from build123d import *

# Parameters (mm, degrees)
SKETCH1_W                              = 14
SKETCH1_H                              = 15
BOSS_EXTRUDE1_DEPTH                    = 50
CBORE_FOR_M6_HEX_HEAD_BOLT1_AT_2_COUNT = 2
CBORE_FOR_M6_HEX_HEAD_BOLT1_AT_2_PITCH = 20


with BuildPart() as part:
    # Sketch1 → Boss-Extrude1 (new body)
    with BuildSketch(Plane.XY):
        Rectangle(SKETCH1_W, SKETCH1_H)
    extrude(amount=BOSS_EXTRUDE1_DEPTH)

    # Sketch3 → CBORE for M6 Hex Head Bolt1 (revolve, cut)
    with BuildSketch(Plane(origin=(-7, 0, 10), x_dir=(0, 0, 1), z_dir=(0, 1, 0))):
        Polygon((0, 0), (0, 14), (3.3, 14), (3.3, 8), (7.2735, 8), (7.2735, 0.025), (7.2985, 0), align=None)
    cbore_for_m6_hex_head_bolt1 = revolve(axis=Axis((-13.35, 0, 10), (1, 0, 0)), mode=Mode.SUBTRACT)

    # CBORE for M6 Hex Head Bolt1 at 2: CBORE for M6 Hex Head Bolt1 ×2
    with Locations(*[(0, 0, i * CBORE_FOR_M6_HEX_HEAD_BOLT1_AT_2_PITCH) for i in range(1, CBORE_FOR_M6_HEX_HEAD_BOLT1_AT_2_COUNT)]):
        add(cbore_for_m6_hex_head_bolt1, mode=Mode.SUBTRACT)


solid = part.part
Can you work these out from the model? Positions are in its coordinate system, mm. A direction names the side the tool comes from. Give positions to 0.01 mm unless a question says otherwise; leave off trailing zeros. Write each loop counter-clockwise with the first axis right and the second up, starting at its lowest first coordinate (ties: lowest second). Pieces come first, ordered by that corner, then holes. Notation, with made-up numbers: M 84,31 L 95,31 A21 cw 95,47 Z; hole C 22,-8 d5. An arc over 180 degrees is marked long. Answer in a Markdown table with one row per item. Add a question column.
Item 1: Imagine slicing it at A-A, the plane y = 0. State how many separate pieces and enclosed holes the cut face has, plus the area to 3 significant figures.
Item 2: We'd pull the mould along Y, two halves only. Please class faces 1 (the flat face through (0, -7.5, 25)), 2 (the cylindrical face through (3.96, 1.26, 33.05)), 3 (the flat face through (0, 0, 50)): released by +Y, released by -Y, zero draft, split by the parting line, or undercut.
Item 3: Please list where these lines run through material, in increasing order: L1, parallel to Z at x = -1.75, y = 0; L2, parallel to Z at x = 5.25, y = 0; L3, parallel to Y at x = 3.75, z = 30.
Item 4: On a 3-axis mill with a long thin cutter (end or side, diameter ignored), from which of +Z, -Z, +X, -X, +Y, -Y can I reach the whole of each face in a straight line? I mean faces 4 (the cylindrical face through (-3.04, -2.18, 36.94)), 5 (the flat face through (0, 0, 0)). Say none if no direction works.
Item 5: For pin 1 Ø8.5 at (y, z) = (0, 10) entering from -X; pin 2 Ø4 at (y, z) = (0, 30) entering from -X, each with a flat end and sliding along its axis, tell me the tip position at first contact or that it passes through.
Item 6: Imagine slicing it at B-B, the plane x = 5.5. Write out the boundary of the cut face in (y, z).
Item 7: Imagine slicing it at D-D, the plane x = -2.25. Write out the boundary of the cut face in (y, z), plus the area to 3 significant figures.
Evaluation:
| question | item | result |
|---|---|---|
| 1 | separate pieces | 3 |
| 1 | enclosed holes | 0 |
| 1 | area | 388 mm² |
| 2 | face 1 | released by -Y |
| 2 | face 2 | undercut |
| 2 | face 3 | zero draft |
| 3 | L1 | z = 0 to 2.73, 17.27 to 22.73, 37.27 to 50 |
| 3 | L2 | z = 0 to 6.7, 13.3 to 26.7, 33.3 to 50 |
| 3 | L3 | y = -7.5 to -3.3, 3.3 to 7.5 |
| 4 | face 4 | -X |
| 4 | face 5 | -Z, +X, -X, +Y, -Y |
| 5 | pin 1 | stops at x = 1 |
| 5 | pin 2 | passes through |
| 6 | outline | M -7.5,0 L 7.5,0 L 7.5,50 L -7.5,50 Z; hole C 0,10 d6.6; hole C 0,30 d6.6 |
| 7 | outline | M -7.5,0 L 7.5,0 L 7.5,50 L -7.5,50 Z; hole C 0,10 d14.55; hole C 0,30 d14.55 |
| 7 | area | 418 mm² |
